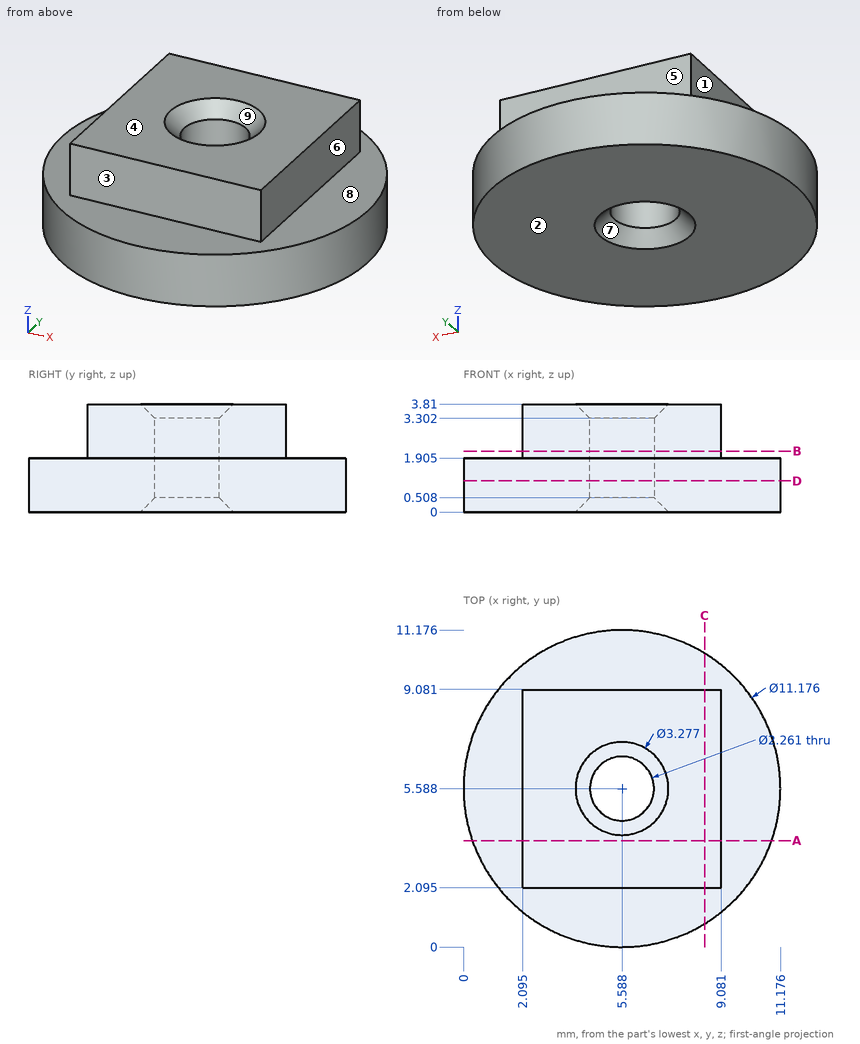
Geometry check sheet. Reference: drawing and pictorial views, mm from the part's lowest x, y, z. A direction names the side the tool comes from. Coordinates: 2 decimals unless noted, no trailing zeros. Order: outer loops, then holes, each group sorted by start corner. A loop starts at its lowest first (then second) coordinate and runs counter-clockwise, first axis right, second up. Notation, with made-up numbers: (-35.75, 75) -> (-12.75, 75) arc R19 cw to (-12.75, 107) -> close; hole circle Ø4 at (37.5, 28.5). An arc over 180 degrees is marked (long way). Write item = value, one per line. Start each with the question number.
1) Cross-section at B-B (z = 2.15). Enter the section's corners in (x, y) (1 decimal).
2) Go/stop test with flat-tipped pins: P1, Ø1, axis at x = 4.5, z = 3, coming from the +Y side; P2, Ø1.5, axis at y = 6, z = 3, coming from the -X side (1 decimal); P3, Ø2, axis at y = 5, z = 3, coming from the +X side. Record where each tip stops, or that it passes through.
3) Cross-section at C-C (x = 8.5). Enter the section's corners in (y, z) (1 decimal), then the cut area to 3 significant figures.
4) Cross-section at D-D (z = 1.1). Enter the section's corners in (x, y) (1 decimal).
5) Mould release check, pull along X, two halves, no side actions. Record for the marked faces 6, 7, 8 and 9: +X half, -X half, draft (parallel to the pull), parting line (faces both ways), or undercut.
6) Cross-section at A-A (y = 3.75). Enter the section's corners in (x, z) (1 decimal).
7) Material ranges on L1, parallel to Y at x = 9, z = 2.4 (1 decimal); L2, parallel to Z at x = 9, y = 9.75 (1 decimal), recorded low to high.
8) Access from +Z, -Z, +X, -X, +Y, -Y to the whole of each face (thin tool, end or side, straight path). Record for the marked faces 1, 2, 3, 4 and 5.
Ans:
q1.outline = (2.1, 2.1) -> (9.1, 2.1) -> (9.1, 9.1) -> (2.1, 9.1) -> close; hole circle Ø2.3 at (5.6, 5.6)
q2.P1 = 9.08
q2.P2 = 2.1
q2.P3 = 9.08
q3.outline = (0.8, 0) -> (10.4, 0) -> (10.4, 1.9) -> (9.1, 1.9) -> (9.1, 3.8) -> (2.1, 3.8) -> (2.1, 1.9) -> (0.8, 1.9) -> close
q3.area = 31.5 mm²
q4.outline = circle Ø11.2 at (5.6, 5.6); hole circle Ø2.3 at (5.6, 5.6)
q5.face_6 = +X half
q5.face_7 = undercut
q5.face_8 = draft
q5.face_9 = undercut
q6.outline = (0.3, 0) -> (10.9, 0) -> (10.9, 1.9) -> (9.1, 1.9) -> (9.1, 3.8) -> (2.1, 3.8) -> (2.1, 1.9) -> (0.3, 1.9) -> close
q7.L1 = 2.1 to 9.1
q7.L2 = 0 to 1.9
q8.face_1 = +Z, -X, +Y, -Y
q8.face_2 = -Z, +X, -X, +Y, -Y
q8.face_3 = +Z, +X, -X, -Y
q8.face_4 = +Z, +X, -X, +Y, -Y
q8.face_5 = +Z, +X, -X, +Y
